For this review, take the finished solid that the model builds, in its own axes (mm). Coordinates: 2 decimals unless noted, no trailing zeros. Loops run counter-clockwise (first coordinate to the right, second up) from the corner with the lowest first, then second, coordinate; pieces in that order, holes last. Notation, with made-up numbers: (62.5, -4.75) -> (89.5, -4.75) arc R20 cw to (89.5, 21.25) -> close; hole circle Ø8 at (-2.75, 61). An arc over 180 degrees is marked (long way). Use a Markdown table: item, result.
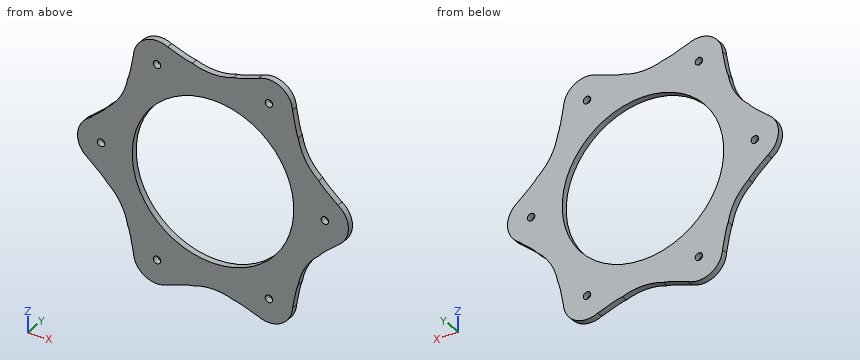
from build123d import *

# Parameters (mm, degrees)
SKETCH1_R           = 45
SKETCH1_R_2         = 32.5
BOSS_EXTRUDE2_DEPTH = 2.5
BOSS_EXTRUDE4_START = -2.5
BOSS_EXTRUDE4_DEPTH = 2.5
CIRPATTERN1_COUNT   = 6
CUT_EXTRUDE2_DEPTH  = 2.5
SKETCH6_R           = 1.5
CUT_EXTRUDE3_DEPTH  = 5


with BuildPart() as part:
    # Sketch1 → Boss-Extrude2 (new body)
    with BuildSketch(Plane(origin=(0, 0, 0), x_dir=(1, 0, 0), z_dir=(0, 1, 0))):
        with Locations(Location((0, 0, 0), (0, 0, 270))):
            Circle(SKETCH1_R)
        with Locations(Location((0, 0, 0), (0, 0, 270))):
            Circle(SKETCH1_R_2, mode=Mode.SUBTRACT)
    extrude(amount=BOSS_EXTRUDE2_DEPTH)

    # Sketch2 → Boss-Extrude4 (add)
    with BuildSketch(Plane(origin=(0, 2.5, 0), x_dir=(1, 0, 0), z_dir=(0, 1, 0)).offset(BOSS_EXTRUDE4_START)):
        with BuildLine():
            ThreePointArc((-42.23454554, 15.532004475), (-45, 0), (-42.23454554, -15.532004475))
            add(Edge.make_bspline(
                [(-50.212380227, -7.942360629), (-45.3159648, -11.95963121), (-42.656686571, -14.489512492), (-42.23454554, -15.532004475)],
                knots=[0.089311832, 0.089311832, 0.089311832, 0.089311832, 1, 1, 1, 1], degree=3))
            ThreePointArc((-50.212380227, -7.942360629), (-54.5, 0), (-50.212380227, 7.942360629))
            add(Edge.make_bspline(
                [(-50.212380227, 7.942360629), (-45.3159648, 11.95963121), (-42.656686571, 14.489512492), (-42.23454554, 15.532004475)],
                knots=[0.089311832, 0.089311832, 0.089311832, 0.089311832, 1, 1, 1, 1], degree=3))
        make_face()
    boss_extrude4 = extrude(amount=BOSS_EXTRUDE4_DEPTH)

    # CirPattern1: Boss-Extrude4 ×6 about axis
    cirpattern1_axis = Axis((0, 2.5, 0), (0, 1, 0))
    for i in range(1, CIRPATTERN1_COUNT):
        add(boss_extrude4.rotate(cirpattern1_axis, i * 360 / CIRPATTERN1_COUNT))

    # Sketch5 → Cut-Extrude2 (cut)
    with BuildSketch(Plane(origin=(0, 2.5, 0), x_dir=(1, 0, 0), z_dir=(0, 1, 0))):
        with BuildLine():
            Line((-8.22468756, 44.342191593), (0, 46.65782144))
            Line((0, 46.65782144), (8.22468756, 44.342191593))
            ThreePointArc((8.22468756, 44.342191593), (0, 42.851652617), (-8.22468756, 44.342191593))
        make_face()
        with BuildLine():
            Line((40.406858652, 23.32891072), (42.513808159, 15.048307431))
            ThreePointArc((42.513808159, 15.048307431), (37.11061976, 21.425826308), (34.289120599, 29.293884161))
            Line((34.289120599, 29.293884161), (40.406858652, 23.32891072))
        make_face()
        with BuildLine():
            Line((40.406858652, -23.32891072), (34.289120599, -29.293884161))
            ThreePointArc((34.289120599, -29.293884161), (37.11061976, -21.425826308), (42.513808159, -15.048307431))
            Line((42.513808159, -15.048307431), (40.406858652, -23.32891072))
        make_face()
        with BuildLine():
            Line((0, -46.65782144), (-8.22468756, -44.342191593))
            ThreePointArc((-8.22468756, -44.342191593), (0, -42.851652617), (8.22468756, -44.342191593))
            Line((8.22468756, -44.342191593), (0, -46.65782144))
        make_face()
        with BuildLine():
            Line((-40.406858652, -23.32891072), (-42.513808159, -15.048307431))
            ThreePointArc((-42.513808159, -15.048307431), (-37.11061976, -21.425826308), (-34.289120599, -29.293884161))
            Line((-34.289120599, -29.293884161), (-40.406858652, -23.32891072))
        make_face()
        with BuildLine():
            Line((-40.406858652, 23.32891072), (-34.289120599, 29.293884161))
            ThreePointArc((-34.289120599, 29.293884161), (-37.11061976, 21.425826308), (-42.513808159, 15.048307431))
            Line((-42.513808159, 15.048307431), (-40.406858652, 23.32891072))
        make_face()
    extrude(amount=-CUT_EXTRUDE2_DEPTH, mode=Mode.SUBTRACT)

    # Sketch6 → Cut-Extrude3 (cut, symmetric)
    with BuildSketch(Plane(origin=(0, 2.5, 0), x_dir=(1, 0, 0), z_dir=(0, 1, 0))):
        with Locations(Location((-45, 0, 0), (0, 0, 270))):
            Circle(SKETCH6_R)
        with Locations(Location((-22.5, 38.97114317, 0), (0, 0, 270))):
            Circle(SKETCH6_R)
        with Locations(Location((22.5, 38.97114317, 0), (0, 0, 270))):
            Circle(SKETCH6_R)
        with Locations(Location((45, 0, 0), (0, 0, 270))):
            Circle(SKETCH6_R)
        with Locations(Location((22.5, -38.97114317, 0), (0, 0, 270))):
            Circle(SKETCH6_R)
        with Locations(Location((-22.5, -38.97114317, 0), (0, 0, 270))):
            Circle(SKETCH6_R)
    extrude(amount=CUT_EXTRUDE3_DEPTH, both=True, mode=Mode.SUBTRACT)


solid = part.part
(1) Take a section at B-B on x = 0. Write out the cut boundary in (y, z), plus the area to 3 significant figures.
Found:
| item | result |
|---|---|
| outline | (0, -42.85) -> (2.5, -42.85) -> (2.5, -32.5) -> (0, -32.5) -> close; (0, 32.5) -> (2.5, 32.5) -> (2.5, 42.85) -> (0, 42.85) -> close |
| area | 51.8 mm^2 |
(2) Take a section at C-C on x = 22.5. Write out the cut boundary in (y, z), plus the area to 3 significant figures.
Found:
| item | result |
|---|---|
| outline | (0, -48.47) -> (2.5, -48.47) -> (2.5, -40.47) -> (0, -40.47) -> close; (0, -37.47) -> (2.5, -37.47) -> (2.5, -23.45) -> (0, -23.45) -> close; (0, 23.45) -> (2.5, 23.45) -> (2.5, 37.47) -> (0, 37.47) -> close; (0, 40.47) -> (2.5, 40.47) -> (2.5, 48.47) -> (0, 48.47) -> close |
| area | 110 mm^2 |
(3) Take a section at D-D on z = 17. Write out the cut boundary in (x, y).
Found:
| item | result |
|---|---|
| outline | (-40.42, 0) -> (-27.7, 0) -> (-27.7, 2.5) -> (-40.42, 2.5) -> close; (27.7, 0) -> (40.42, 0) -> (40.42, 2.5) -> (27.7, 2.5) -> close |
(4) For line 1 along X through (y, z) = (1.65, 0); line 2 along X through (y, z) = (1.45, 13); line 3 along X through (y, z) = (1.7, -7), list the stretches that pass through material, from the lowest coordinate up.
Found:
| item | result |
|---|---|
| line 1 | x = -54.5 to -46.5, -43.5 to -32.5, 32.5 to 43.5, 46.5 to 54.5 |
| line 2 | x = -44.39 to -29.79, 29.79 to 44.39 |
| line 3 | x = -51.42 to -31.74, 31.74 to 51.42 |
(5) For pin 1 Ø1.5 at (x, y) = (-21, 1.5) entering from +Z; pin 2 Ø1.5 at (x, y) = (27, 1) entering from +Z; pin 3 Ø10 at (x, z) = (38.5, 38) entering from -Y; pin 4 Ø1.5 at (y, z) = (1, -34.5) entering from +X, all flat-tipped, find the tip position at first contact; note any pin that passes through.
Found:
| item | result |
|---|---|
| pin 1 | stops at z = 48.44 |
| pin 2 | stops at z = 47.7 |
| pin 3 | passes through |
| pin 4 | stops at x = 33.04 |
(6) Take a section at A-A on z = 0. Write out the cut boundary in (x, y), plus the area to 3 significant figures.
Found:
| item | result |
|---|---|
| outline | (-54.5, 0) -> (-46.5, 0) -> (-46.5, 2.5) -> (-54.5, 2.5) -> close; (-43.5, 0) -> (-32.5, 0) -> (-32.5, 2.5) -> (-43.5, 2.5) -> close; (32.5, 0) -> (43.5, 0) -> (43.5, 2.5) -> (32.5, 2.5) -> close; (46.5, 0) -> (54.5, 0) -> (54.5, 2.5) -> (46.5, 2.5) -> close |
| area | 95.0 mm^2 |
